Here's how the part is built. I have some questions about the finished solid (model axes, mm). A direction names the side the tool comes from. Round coordinates to 2 decimals unless told otherwise and drop trailing zeros. Order: outer loops, then holes, each group sorted by start corner. A loop starts at its lowest first (then second) coordinate and runs counter-clockwise, first axis right, second up. Notation, with made-up numbers: (-17.75, 30) -> (18.25, 30) arc R21 cw to (18.25, 36) -> close; hole circle Ø10 at (61.25, 36). An arc over 180 degrees is marked (long way). One line per item, written item: value.
```python
from build123d import *

# Parameters (mm, degrees)
BOSS_EXTRUDE1_DEPTH     = 63.399999946
BOSS_EXTRUDE2_DEPTH     = 63.399999946
BOSS_EXTRUDE3_DEPTH     = 5
BOSS_EXTRUDE4_DEPTH     = 2.5
SKETCH8_W               = 50.000000076
SKETCH8_H               = 34.99999985
CUT_EXTRUDE2_DEPTH      = 12.5
CUT_EXTRUDE4_DEPTH      = 2.5
SKETCH10_W              = 9.999999939
SKETCH10_H              = 34.99999985
CUT_EXTRUDE5_DEPTH      = 2.5
BOSS_EXTRUDE6_DEPTH     = 58.399999946
BOSS_EXTRUDE7_DEPTH     = 63.399999946
CUT_EXTRUDE8_DEPTH      = 633.390638366
CUT_EXTRUDE8_DEPTH_BACK = 633.390638366
SKETCH13_R              = 207.367939984
CUT_EXTRUDE9_DEPTH      = 465.722133037
BOSS_EXTRUDE15_DEPTH    = 63.4


with BuildPart() as part:
    # Sketch1 → Boss-Extrude1 (new body)
    with BuildSketch(Plane(origin=(0, 0, 0), x_dir=(1, 0, 0), z_dir=(0, 1, 0))):
        Polygon((-304.507375635, 63.663075045), (-304.507375635, -102.743315535), (-191.856739857, -143.33813924), (108.841988943, -143.33813924), (221.492624721, -102.743315535), (221.492624721, 63.663075045), (218.992624721, 63.663075045), (218.992624721, -100.986845182), (108.405283491, -140.83813932), (-191.420034405, -140.83813932), (-302.007375635, -100.986845182), (-302.007375635, 63.663075045), align=None)
    extrude(amount=BOSS_EXTRUDE1_DEPTH)



with BuildPart() as body_2:
    # Sketch3 → Boss-Extrude2 (new body)
    with BuildSketch(Plane(origin=(0, 0, 0), x_dir=(1, 0, 0), z_dir=(0, 1, 0))):
        Polygon((-304.507375635, 179.416332489), (-159.011838483, 344.817501188), (75.997087569, 344.817501188), (221.492624721, 179.416332489), (221.492624721, 63.663075045), (218.992624721, 63.663075045), (218.992624721, 178.473242754), (74.866627441, 342.317501188), (-157.881378355, 342.317501188), (-302.007375635, 178.473242754), (-302.007375635, 63.663075045), (-304.507375635, 63.663075045), align=None)
    extrude(amount=BOSS_EXTRUDE2_DEPTH)


with BuildPart() as part_1:
    add(part.part)

    add(body_2.part)  # Boss-Extrude3 merges body 2
    # Sketch5 → Boss-Extrude3 (add)
    with BuildSketch(Plane(origin=(0, 0, 0), x_dir=(1, 0, 0), z_dir=(0, 1, 0))):
        Polygon((208.992624721, 174.700883815), (208.992624721, 63.663075045), (218.992624721, 63.663075045), (218.992624721, 178.473242754), (74.866627441, 342.317501188), (-157.881378355, 342.317501188), (-302.007375635, 178.473242754), (-302.007375635, 63.663075045), (-292.007375635, 63.663075045), (-292.007375635, 174.700883815), (-153.359537842, 332.317501188), (70.344786927, 332.317501188), align=None)
        Polygon((215.602428975, -91.579051987), (106.658461628, -130.83813932), (-189.673212543, -130.83813932), (-298.617179889, -91.579051987), (-302.007375635, -100.986845182), (-191.420034405, -140.83813932), (108.405283491, -140.83813932), (218.992624721, -100.986845182), align=None)
    extrude(amount=BOSS_EXTRUDE3_DEPTH)

    # Sketch6 → Boss-Extrude4 (add)
    with BuildSketch(Plane(origin=(0, 63.399999946, 0), x_dir=(1, 0, 0), z_dir=(0, 1, 0))):
        Polygon((-159.011838483, 344.817501188), (-304.507375635, 179.416332489), (-304.507375635, -102.743315535), (-191.856739857, -143.33813924), (108.841988943, -143.33813924), (221.492624721, -102.743315535), (221.492624721, 179.416332489), (75.997087569, 344.817501188), align=None)
    extrude(amount=BOSS_EXTRUDE4_DEPTH)

    # Sketch8 → Cut-Extrude2 (cut)
    with BuildSketch(Plane(origin=(0, 0, -344.817501188), x_dir=(-1, 0, 0), z_dir=(0, 0, -1))):
        Polygon((6.50737548, 28.400000096), (6.50737548, 0), (76.507375434, 0), (76.507375434, 28.400000096), (66.507375495, 28.400000096), (16.507375419, 28.400000096), align=None)
        with Locations((41.507375457, 45.900000021)):
            Rectangle(SKETCH8_W, SKETCH8_H)
    extrude(amount=-CUT_EXTRUDE2_DEPTH, mode=Mode.SUBTRACT)

    # Sketch9 → Cut-Extrude4 (cut)
    with BuildSketch(Plane(origin=(0, 65.899999946, 0), x_dir=(1, 0, 0), z_dir=(0, 1, 0))):
        with BuildLine():
            ThreePointArc((-76.507375434, 344.817501188), (-41.507375457, 309.817501211), (-6.50737548, 344.817501188))
            Line((-6.50737548, 344.817501188), (-16.507375419, 344.817501188))
            Line((-16.507375419, 344.817501188), (-66.507375495, 344.817501188))
            Line((-66.507375495, 344.817501188), (-76.507375434, 344.817501188))
        make_face()
        with BuildLine():
            Line((-16.507375419, 344.817501188), (-6.50737548, 344.817501188))
            ThreePointArc((-6.50737548, 344.817501188), (-41.507375457, 379.817501165), (-76.507375434, 344.817501188))
            Line((-76.507375434, 344.817501188), (-66.507375495, 344.817501188))
            Line((-66.507375495, 344.817501188), (-16.507375419, 344.817501188))
        make_face()
    extrude(amount=-CUT_EXTRUDE4_DEPTH, mode=Mode.SUBTRACT)

    # Sketch10 → Cut-Extrude5 (cut)
    with BuildSketch(Plane(origin=(0, 0, -344.817501188), x_dir=(-1, 0, 0), z_dir=(0, 0, -1))):
        with Locations((11.50737545, 45.900000021)):
            Rectangle(SKETCH10_W, SKETCH10_H)
        with Locations((71.507375465, 45.900000021)):
            Rectangle(SKETCH10_W, SKETCH10_H)
    extrude(amount=-CUT_EXTRUDE5_DEPTH, mode=Mode.SUBTRACT)

    # Sketch11 → Boss-Extrude6 (add)
    with BuildSketch(Plane(origin=(0, 5, 0), x_dir=(1, 0, 0), z_dir=(0, 1, 0))):
        Polygon((-76.507375434, 332.317501188), (-76.507375434, 342.317501188), (-157.881378355, 342.317501188), (-302.007375635, 178.473242754), (-302.007375635, 63.663075045), (-292.007375635, 63.663075045), (-292.007375635, 174.700883815), (-153.359537842, 332.317501188), align=None)
        Polygon((208.992624721, 63.663075045), (218.992624721, 63.663075045), (218.992624721, 178.473242754), (74.866627441, 342.317501188), (-6.50737548, 342.317501188), (-6.50737548, 332.317501188), (70.344786927, 332.317501188), (208.992624721, 174.700883815), align=None)
        Polygon((108.405283491, -140.83813932), (218.992624721, -100.986845182), (215.602428975, -91.579051987), (106.658461628, -130.83813932), (-189.673212543, -130.83813932), (-298.617179889, -91.579051987), (-302.007375635, -100.986845182), (-191.420034405, -140.83813932), align=None)
    extrude(amount=BOSS_EXTRUDE6_DEPTH)

    # Sketch12 → Boss-Extrude7 (add)
    with BuildSketch(Plane.XZ):
        Polygon((-302.007375635, 100.986845182), (-302.007375635, -63.663075045), (-292.007375635, -63.663075045), (-292.007375635, 93.96096343), (-298.617179889, 91.579051987), align=None)
        Polygon((218.992624721, 100.986845182), (218.992624721, -63.663075045), (208.992624721, -63.663075045), (208.992624721, 93.96096343), (215.602428975, 91.579051987), align=None)
    extrude(amount=-BOSS_EXTRUDE7_DEPTH)

    # Sketch2 → Cut-Extrude8 (cut, two sides: drawn at the far end of the back side and taken through both)
    with BuildSketch(Plane.ZY.offset(304.507375635).offset(-CUT_EXTRUDE8_DEPTH_BACK)):
        with BuildLine():
            ThreePointArc((-63.663075045, 0), (-22.645494652, -138.842602216), (95.238139156, -54.800000095))
            ThreePointArc((95.238139156, -54.800000095), (90.380741277, -25.816366286), (76.339353357, 0))
            Line((76.339353357, 0), (-63.663075045, 0))
        make_face()
        with BuildLine():
            Line((-63.663075045, 0), (76.339353357, 0))
            ThreePointArc((76.339353357, 0), (6.338139156, 34.099999905), (-63.663075045, 0))
        make_face()
    extrude(amount=CUT_EXTRUDE8_DEPTH + CUT_EXTRUDE8_DEPTH_BACK, mode=Mode.SUBTRACT)

    # Sketch13 → Cut-Extrude9 (cut, through all)
    with BuildSketch(Plane(origin=(0, 65.899999946, 0), x_dir=(1, 0, 0), z_dir=(0, 1, 0))):
        with Locations((-41.507375457, 127.449561204)):
            Circle(SKETCH13_R)
    extrude(amount=-CUT_EXTRUDE9_DEPTH, mode=Mode.SUBTRACT)

    # Sketch16 → Boss-Extrude15 (add, through all)
    with BuildSketch(Plane.XZ.offset(-63.399999946)):
        with BuildLine():
            Line((-292.007375635, -174.700883815), (-243.420166148, -174.700883815))
            ThreePointArc((-243.420166148, -174.700883815), (-244.727222578, -168.718875101), (-245.857092333, -162.700883815))
            Line((-245.857092333, -162.700883815), (-292.007375635, -162.700883815))
            Line((-292.007375635, -162.700883815), (-292.007375635, -174.700883815))
        make_face()
        with BuildLine():
            Line((-292.007375635, -66.656438986), (-239.763923455, -66.656438986))
            ThreePointArc((-239.763923455, -66.656438986), (-241.223768745, -71.638945859), (-242.558416908, -76.656438986))
            Line((-242.558416908, -76.656438986), (-292.007375635, -76.656438986))
            Line((-292.007375635, -76.656438986), (-292.007375635, -66.656438986))
        make_face()
        with BuildLine():
            Line((-223.513560978, 118.643419163), (-223.513560978, -28.075465156))
            ThreePointArc((-223.513560978, -28.075465156), (-214.696000108, -13.400611956), (-204.697974588, 0.496876373))
            Line((-204.697974588, 0.496876373), (-204.697974588, 125.423810655))
            Line((-204.697974588, 125.423810655), (-223.513560978, 118.643419163))
        make_face()
        with BuildLine():
            Line((-189.673212543, 130.83813932), (-189.673212543, 17.63092423))
            ThreePointArc((-189.673212543, 17.63092423), (-182.344298329, 24.755641365), (-174.673212543, 31.510567025))
            Line((-174.673212543, 31.510567025), (-174.673212543, 115.83813932))
            Line((-174.673212543, 115.83813932), (91.658461628, 115.83813932))
            Line((91.658461628, 115.83813932), (91.658461628, 31.510567025))
            ThreePointArc((91.658461628, 31.510567025), (99.329547415, 24.755641365), (106.658461628, 17.63092423))
            Line((106.658461628, 17.63092423), (106.658461628, 130.83813932))
            Line((106.658461628, 130.83813932), (-189.673212543, 130.83813932))
        make_face()
        with BuildLine():
            Line((121.683223673, 125.423810655), (121.683223673, 0.496876373))
            ThreePointArc((121.683223673, 0.496876373), (131.681249194, -13.400611956), (140.498810064, -28.075465156))
            Line((140.498810064, -28.075465156), (140.498810064, 118.643419163))
            Line((140.498810064, 118.643419163), (121.683223673, 125.423810655))
        make_face()
        with BuildLine():
            Line((208.992624721, -66.656438986), (156.749172541, -66.656438986))
            ThreePointArc((156.749172541, -66.656438986), (158.115408542, -71.30504552), (159.372662829, -75.984303492))
            Line((159.372662829, -75.984303492), (208.992624721, -75.984303492))
            Line((208.992624721, -75.984303492), (208.992624721, -66.656438986))
        make_face()
        with BuildLine():
            Line((208.992624721, -174.700883815), (160.405415234, -174.700883815))
            ThreePointArc((160.405415234, -174.700883815), (161.712471663, -168.718875101), (162.842341419, -162.700883815))
            Line((162.842341419, -162.700883815), (208.992624721, -162.700883815))
            Line((208.992624721, -162.700883815), (208.992624721, -174.700883815))
        make_face()
    extrude(amount=BOSS_EXTRUDE15_DEPTH)


solid = part_1.part
```
Q1. I want a section at A-A on z = -311.5. Write out the boundary of the cut face in (x, y).
Answers:
outline: (-188.32, 0) -> (-171.67, 0) -> (-171.67, 63.4) -> (-137.04, 63.4) -> (-137.04, 65.9) -> (-188.32, 65.9) -> close; (54.03, 63.4) -> (88.66, 63.4) -> (88.66, 0) -> (105.3, 0) -> (105.3, 65.9) -> (54.03, 65.9) -> close
Q2. I want a section at D-D on x = -216. Write out the boundary of the cut face in (y, z), then the cut area to 3 significant figures.
Answers:
outline: (0, -280.03) -> (65.9, -280.03) -> (65.9, -239.49) -> (63.4, -239.49) -> (63.4, -261.11) -> (0, -261.11) -> close; (0, -15.41) -> (65.9, -15.41) -> (65.9, 134.64) -> (0, 134.64) -> close
area: 11,200 mm2
Q3. I need wall thicknesses on line 1 along X through (y, z) = (60, 4); line 2 along Z through (x, y) = (16, 18); line 3 along X through (y, z) = (10.5, -59). Which ranges of each line are inside material? Lowest first, please.
Answers:
line 1: -304.51 to -292.01, -223.51 to -204.7, 121.68 to 140.5, 208.99 to 221.49
line 2: -344.82 to -332.32, 115.84 to 143.34
line 3: -304.51 to -292.01, 208.99 to 221.49
Q4. If we mould it in two halves opening along X, with no side actions, what happens to faces 4 (the face through (-304.507, 40, -40)), 5 (the face through (184, 32, -75.984)), 6 (the face through (-259, 0, -214))? For each: pulls with the +X half, pulls with the -X half, needs draft (parallel to the pull), parting line crosses it, or undercut.
Answers:
face 4: pulls with the -X half
face 5: undercut
face 6: needs draft
Q5. For P1, Ø4.5, axis at x = -201, z = 58, coming from the -Y side; P2, Ø23, axis at x = -271.5, y = 17, coming from the +Z side; P3, Ø3, axis at y = 28, z = 34, coming from the -X side; P4, Ø12, axis at x = 156, z = -150.5, coming from the -Y side, each with a flat end and sliding along its axis, tell me the tip position at first contact or that it passes through.
Answers:
P1: y = 63.4
P2: z = 118.78
P3: x = -223.51
P4: through
Q6. Which directions (+Z, -Z, +X, -X, +Y, -Y) give clear straight access to the entire face, cutting with the end or side of a thin tool? Please do faces 1 (the face through (-204.698, 32, 62)), 2 (the face through (-117, 32, -344.818)), 3 (the face through (-76.507, 31, -338)).
Answers:
face 1: -Y
face 2: -Z, +X, -X, +Y, -Y
face 3: -Z, -Y
Q7. I want a section at B-B on x = 19. Write out the boundary of the cut face in (y, z), then the cut area to 3 significant figures.
Answers:
outline: (0, -344.82) -> (65.9, -344.82) -> (65.9, -325.79) -> (63.4, -325.79) -> (63.4, -332.32) -> (0, -332.32) -> close; (0, 115.84) -> (63.4, 115.84) -> (63.4, 70.89) -> (65.9, 70.89) -> (65.9, 143.34) -> (0, 143.34) -> close
area: 2,760 mm2
Q8. I want a section at C-C on y = 10.5. Give the number of separate pieces and of enclosed holes in the cut face, then the cut area to 3 significant figures.
Answers:
separate pieces: 3
enclosed holes: 0
area: 32,200 mm2
